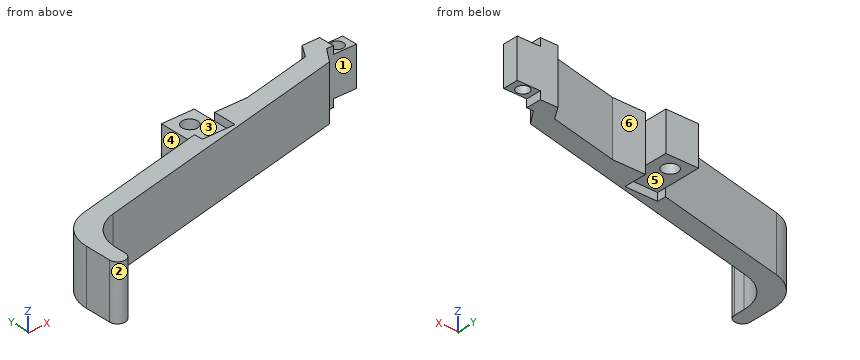
```python
from build123d import *

# Parameters (mm, degrees)
BOSS_EXTRUDE2_DEPTH = 7
BOSS_EXTRUDE3_DEPTH = 7
SKETCH3_R           = 1
CUT_EXTRUDE1_DEPTH  = 7
SKETCH4_R           = 0.8
CUT_EXTRUDE2_DEPTH  = 7
SKETCH6_W           = 2.954985002
SKETCH6_H           = 1
CUT_EXTRUDE3_DEPTH  = 10
SKETCH7_W           = 4.187886823
SKETCH7_H           = 1
CUT_EXTRUDE5_DEPTH  = 6


with BuildPart() as part:
    # Sketch1 → Boss-Extrude2 (new body)
    with BuildSketch(Plane.XY):
        with BuildLine():
            Line((3.153391707, 12.247099593), (4.296460399, 14.043350396))
            Line((4.296460399, 14.043350396), (9.489380334, 14.043350396))
            Line((9.489380334, 14.043350396), (9.489380334, 12.043350396))
            Line((9.489380334, 12.043350396), (5.687282028, 12.043350396))
            Line((5.687282028, 12.043350396), (4.296460399, 10.01751105))
            Line((4.296460399, 10.01751105), (-29.974468214, 2.361481073))
            ThreePointArc((-29.974468214, 2.361481073), (-32.786312372, 0.608216504), (-33.884352793, -2.51823699))
            Line((-33.884352793, -2.51823699), (-33.884352793, -3.909471954))
            ThreePointArc((-33.884352793, -3.909471954), (-34.884352793, -4.909471954), (-35.884352793, -3.909471954))
            Line((-35.884352793, -3.909471954), (-35.884352793, -0.480084513))
            ThreePointArc((-35.884352793, -0.480084513), (-34.786312372, 2.646368981), (-31.974468214, 4.399633549))
            Line((-31.974468214, 4.399633549), (3.153391707, 12.247099593))
        make_face()
    extrude(amount=BOSS_EXTRUDE2_DEPTH)

    # Sketch2 → Boss-Extrude3 (add)
    with BuildSketch(Plane.XY.offset(7)):
        Polygon((-6.034764609, 10.194491069), (-10.222651431, 10.194491069), (-10.222651431, 13.1883213), (-14.410538254, 13.1883213), (-14.410538254, 10.194491069), (-14.410538254, 8.323366571), align=None)
    extrude(amount=-BOSS_EXTRUDE3_DEPTH)

    # Sketch3 → Cut-Extrude1 (cut)
    with BuildSketch(Plane.XY.offset(7)):
        with Locations((-12.414768406, 11.299883581)):
            Circle(SKETCH3_R)
    extrude(amount=-CUT_EXTRUDE1_DEPTH, mode=Mode.SUBTRACT)

    # Sketch4 → Cut-Extrude2 (cut)
    with BuildSketch(Plane.XY.offset(7)):
        with Locations((7.932339973, 13.090243395)):
            Circle(SKETCH4_R)
    extrude(amount=-CUT_EXTRUDE2_DEPTH, mode=Mode.SUBTRACT)

    # Sketch6 → Cut-Extrude3 (cut)
    with BuildSketch(Plane.XZ.offset(-12.043350396)):
        with Locations((8.011887833, 6.5)):
            Rectangle(SKETCH6_W, SKETCH6_H)
        with Locations((8.011887833, 0.5)):
            Rectangle(SKETCH6_W, SKETCH6_H)
    extrude(amount=-CUT_EXTRUDE3_DEPTH, mode=Mode.SUBTRACT)

    # Sketch7 → Cut-Extrude5 (cut)
    with BuildSketch(Plane(origin=(0, 13.1883213, 0), x_dir=(1, 0, 0), z_dir=(0, 1, 0))):
        with Locations((-12.316594843, -0.5)):
            Rectangle(SKETCH7_W, SKETCH7_H)
        with Locations((-12.316594843, -6.5)):
            Rectangle(SKETCH7_W, SKETCH7_H)
    extrude(amount=-CUT_EXTRUDE5_DEPTH, mode=Mode.SUBTRACT)


solid = part.part
```
Part model, mm, in its own coordinate system. Face numbers are marked on the shaded views. A direction names the side the tool comes from. Round coordinates to 2 decimals unless told otherwise and drop trailing zeros. Write each loop counter-clockwise with the first axis right and the second up, starting at its lowest first coordinate (ties: lowest second). Pieces come first, ordered by that corner, then holes. Notation, with made-up numbers: (16.5, 71.25) -> (24.5, 71.25) arc R27 ccw to (24.5, 87.25) -> close; hole circle Ø10 at (10, 59). An arc over 180 degrees is marked (long way). Return JSON: item names as keys, results as strings. Group by question number.
Q1. Saw through at D-D on y = -3.5. Write the cut outline in (x, z), plus the area to 3 significant figures.
Q2. Probe L1, parallel to X at y = -3.5, z = 3.25; L2, parallel to Y at x = 7, z = 1.5; L3, parallel to X at y = 13.5, z = 5. List the from-to ranges inside material, lowest first. Write a range as [from, to].
Q3. Saw through at C-C on x = 5. Write the cut outline in (y, z), plus the area to 3 significant figures.
Q4. Mould opens along X. For the marked faces 1, 2 and 3 say: pulls with the +X half, pulls with the -X half, needs draft (parallel to the pull), parting line crosses it, or undercut.
Q5. Which spindle directions (+Z, -Z, +X, -X, +Y, -Y) get a long thin tool onto all of the face, cutting with end or side? Do the marked faces 4, 5 and 6. Say none if no direction does.
Q6. Saw through at B-B on y = 9. Write the cut outline in (x, z), plus the area to 3 significant figures.
Q7. Pin check, flat tips, straight feed: pin 1 (1.9 mm diameter, centred on x = 7, z = 3, fed in from -Y); pin 2 (3.5 mm diameter, centred on x = -12.5, y = 10.5, fed in from +Z); pin 3 (0.8 mm diameter, centred on y = 9, z = 6.5, fed in from -X). Stop position of each tip, or through.
Q8. Saw through at A-A on z = 6.5. Write the cut outline in (x, y), plus the area to 3 significant figures.
Answer:
{
 "1": {"outline": "(-35.88, 0) -> (-33.88, 0) -> (-33.88, 7) -> (-35.88, 7) -> close", "area": "14.0 mm2"},
 "2": {"L1": "[-35.88, -33.88]", "L2": "[12.04, 14.04]", "L3": "[3.95, 7.25], [8.62, 9.49]"},
 "3": {"outline": "(11.04, 0) -> (14.04, 0) -> (14.04, 7) -> (11.04, 7) -> close", "area": "21.0 mm2"},
 "4": {"face 1": "needs draft", "face 2": "parting line crosses it", "face 3": "undercut"},
 "5": {"face 4": "+Z, -Z, -X, +Y", "face 5": "-Z, +Y", "face 6": "+Z, -Z, +Y"},
 "6": {"outline": "(-14.41, 1) -> (-10.22, 1) -> (-10.22, 0) -> (-0.26, 0) -> (-0.26, 7) -> (-10.22, 7) -> (-10.22, 6) -> (-14.41, 6) -> close", "area": "90.7 mm2"},
 "7": {"pin 1": "y = 12.04", "pin 2": "z = 6", "pin 3": "x = -10.22"},
 "8": {"outline": "(-35.88, -3.91) arc R1 ccw to (-33.88, -3.91) -> (-33.88, -2.52) arc R5 cw to (-29.97, 2.36) -> (4.3, 10.02) -> (5.69, 12.04) -> (6.53, 12.04) -> (6.53, 14.04) -> (4.3, 14.04) -> (3.15, 12.25) -> (-6.03, 10.19) -> (-10.22, 10.19) -> (-10.22, 7.19) -> (-14.41, 7.19) -> (-14.41, 8.32) -> (-31.97, 4.4) arc R5 ccw to (-35.88, -0.48) -> close", "area": "114 mm2"}
}
